Geometry check sheet. Reference: the model listing, model coordinates, mm. Give positions to 0.01 mm unless a question says otherwise; leave off trailing zeros. Order: outer loops, then holes, each group sorted by start corner. A loop starts at its lowest first (then second) coordinate and runs counter-clockwise, first axis right, second up.
from build123d import *

# Parameters (mm, degrees)
CYLINDER001_R          = 0.3
CYLINDER001_DEPTH      = 10
CYLINDER002_R          = 0.3
CYLINDER002_DEPTH      = 10
CYLINDER_R             = 6
CYLINDER_DEPTH         = 4.5
FILLET_R               = 2.2
FILLET_PITCH_ANGLE     = -90
FILLET_PLACEMENT_ANGLE = 90


with BuildPart() as pin1:
    # Cylinder001 → Cylinder001 (new body)
    with BuildSketch(Plane(origin=(-3.75, 0, -3), x_dir=(1, 0, 0), z_dir=(0, 0, 1))):
        Circle(CYLINDER001_R)
    extrude(amount=CYLINDER001_DEPTH)


with BuildPart() as pin2:
    # Cylinder002 → Cylinder002 (new body)
    with BuildSketch(Plane(origin=(3.75, 0, -3), x_dir=(1, 0, 0), z_dir=(0, 0, 1))):
        Circle(CYLINDER002_R)
    extrude(amount=CYLINDER002_DEPTH)


with BuildPart() as fusion:
    # Cylinder → Cylinder (new body)
    with BuildSketch(Plane.XY):
        Circle(CYLINDER_R)
    extrude(amount=CYLINDER_DEPTH)

    # Fillet
    fillet_edges = [fusion.edges().sort_by_distance(p)[0] for p in [
        (-6, 0, 4.5),
        (-6, 0, 0),
    ]]
    fillet(fillet_edges, radius=FILLET_R)


with BuildPart() as fusion_1:
    # Fillet pitch: moved
    add(fusion.part.rotate(Axis((0, 0, 0), (0, 1, 0)), FILLET_PITCH_ANGLE))


with BuildPart() as fusion_2:
    # Fillet placement: moved
    add(fusion_1.part.moved(Location((0, 2.25, 9))).rotate(Axis((0, 2.25, 9), (0, 0, 1)), FILLET_PLACEMENT_ANGLE))

    # Fusion: union Pin1, Pin2
    add(pin1.part)
    add(pin2.part)


solid = fusion_2.part
Item 1: Sectioned sample at D-D (z = 3.75). Give the number of separate pieces and of enclosed holes in the cut face, and give its area (3 significant figures).
Reported:
separate pieces: 3
enclosed holes: 0
area: 16.5 mm2
Item 2: Sectioned sample at C-C (y = 0.65). Enter the section's corners in (x, z), and give its area (3 significant figures).
Reported:
outline: circle Ø11.83 at (0, 9)
area: 110 mm2
Item 3: Sectioned sample at A-A (z = 1). Enter the section's corners in (x, y), and give its area (3 significant figures).
Reported:
outline: circle Ø0.6 at (-3.75, 0); circle Ø0.6 at (3.75, 0)
area: 0.565 mm2
Item 4: Gauge pin test, flat ends, axial feed: pin 1 (2 mm diameter, centred on x = -0.5, y = 0.5, fed in from -Z); pin 2 (6 mm diameter, centred on x = 2, z = 5.5, fed in from -Y). Record the tip position at first contact, or that the pin passes through.
Reported:
pin 1: stops at z = 3
pin 2: stops at y = -2.25
Item 5: Scan lines: L1, parallel to Y at x = 3.75, z = 3.5; L2, parallel to X at y = 0.1, z = -0.25; L3, parallel to X at y = 1.75, z = 12.75. Record each from-to range of solid material in increasing order.
Reported:
L1: y = -0.3 to 0.3
L2: x = -4.03 to -3.47, 3.47 to 4.03
L3: x = -3.6 to 3.6
Item 6: Sectioned sample at B-B (x = 0). Enter the section's corners in (y, z).
Reported:
outline: (-2.25, 5.2) arc R2.2 ccw to (-0.05, 3) - (0.05, 3) arc R2.2 ccw to (2.25, 5.2) - (2.25, 12.8) arc R2.2 ccw to (0.05, 15) - (-0.05, 15) arc R2.2 ccw to (-2.25, 12.8) - close
